```python
from build123d import *

# Parameters (mm, degrees)
SKETCH1_R           = 1.35
BOSS_EXTRUDE1_DEPTH = 3
SKETCH2_R           = 2
CUT_EXTRUDE1_DEPTH  = 110.604839186
FILLET1_R           = 2


with BuildPart() as part:
    # Sketch1 → Boss-Extrude1 (new body)
    with BuildSketch(Plane.XY):
        Polygon((78.713203436, 49.493203436), (57.5, 28.28), (57.5, -28.28), (78.713203436, -49.493203436), (51.993203436, -76.213203436), (30.78, -55), (-30.78, -55), (-51.993203436, -76.213203436), (-78.713203436, -49.493203436), (-57.5, -28.28), (-57.5, 28.28), (-78.713203436, 49.493203436), (-51.993203436, 76.213203436), (-30.78, 55), (30.78, 55), (51.993203436, 76.213203436), align=None)
        with Locations((29, -24.5)):
            Circle(SKETCH1_R, mode=Mode.SUBTRACT)
        with Locations((29, 24.5)):
            Circle(SKETCH1_R, mode=Mode.SUBTRACT)
        with Locations((-29, -24.5)):
            Circle(SKETCH1_R, mode=Mode.SUBTRACT)
        with Locations((-29, 24.5)):
            Circle(SKETCH1_R, mode=Mode.SUBTRACT)
    extrude(amount=BOSS_EXTRUDE1_DEPTH)

    # Sketch2 → Cut-Extrude1 (cut, through all)
    with BuildSketch(Plane.XY.offset(3)):
        with Locations((43.079339828, 53.30726189)):
            Circle(SKETCH2_R)
        with Locations((53.685941546, 63.913863607)):
            Circle(SKETCH2_R)
        with Locations((55.80726189, 40.579339828)):
            Circle(SKETCH2_R)
        with Locations((66.413863607, 51.185941546)):
            Circle(SKETCH2_R)
        with Locations((-66.413863607, -51.185941546)):
            Circle(SKETCH2_R)
        with Locations((-55.80726189, -40.579339828)):
            Circle(SKETCH2_R)
        with Locations((-43.079339828, -53.30726189)):
            Circle(SKETCH2_R)
        with Locations((-53.685941546, -63.913863607)):
            Circle(SKETCH2_R)
        with Locations((-53.479114875, 64.120690278)):
            Circle(SKETCH2_R)
        with Locations((-42.872513158, 53.51408856)):
            Circle(SKETCH2_R)
        with Locations((-55.600435219, 40.786166499)):
            Circle(SKETCH2_R)
        with Locations((-66.207036937, 51.392768217)):
            Circle(SKETCH2_R)
        with Locations((55.600435219, -40.786166499)):
            Circle(SKETCH2_R)
        with Locations((42.872513157, -53.51408856)):
            Circle(SKETCH2_R)
        with Locations((66.207036937, -51.392768217)):
            Circle(SKETCH2_R)
        with Locations((53.479114875, -64.120690278)):
            Circle(SKETCH2_R)
        with BuildLine():
            Line((-38.5, 17.5), (-38.5, -17.5))
            ThreePointArc((-38.5, -17.5), (-45.5, -24.5), (-52.5, -17.5))
            Line((-52.5, -17.5), (-52.5, 17.5))
            ThreePointArc((-52.5, 17.5), (-45.5, 24.5), (-38.5, 17.5))
        make_face()
        with BuildLine():
            Line((38.5, 17.5), (38.5, -17.5))
            ThreePointArc((38.5, -17.5), (45.5, -24.5), (52.5, -17.5))
            Line((52.5, -17.5), (52.5, 17.5))
            ThreePointArc((52.5, 17.5), (45.5, 24.5), (38.5, 17.5))
        make_face()
    extrude(amount=-CUT_EXTRUDE1_DEPTH, mode=Mode.SUBTRACT)

    # Fillet1
    fillet1_edges = [part.edges().sort_by_distance(p)[0] for p in [
        (78.713203436, -49.493203436, 1.5),
        (51.993203436, -76.213203436, 1.5),
        (-51.993203436, -76.213203436, 1.5),
        (-78.713203436, -49.493203436, 1.5),
        (-78.713203436, 49.493203436, 1.5),
        (-51.993203436, 76.213203436, 1.5),
        (51.993203436, 76.213203436, 1.5),
        (78.713203436, 49.493203436, 1.5),
    ]]
    fillet(fillet1_edges, radius=FILLET1_R)


solid = part.part
```
Can you work these out from the model? Positions are in its coordinate system, mm. A direction names the side the tool comes from. Round coordinates to 2 decimals unless told otherwise and drop trailing zeros. Loops run counter-clockwise (first coordinate to the right, second up) from the corner with the lowest first, then second, coordinate; pieces in that order, holes last. Notation, with made-up numbers: M 88.5,66.25 L 112.5,66.25 A25 cw 112.5,86.25 Z; hole C 4,22 d5. An arc over 180 degrees is marked long. Answer as a JSON object with one key per item and string values. Group by question number.
Q1. Imagine slicing it at A-A, the plane y = 1. Please give me the cut outline in (x, z), then the cut area to 3 significant figures.
Q2. Imagine slicing it at B-B, the plane x = 6.5. Please give me the cut outline in (y, z), then the cut area to 3 significant figures.
Q3. On a 3-axis mill with a long thin cutter (end or side, diameter ignored), from which of +Z, -Z, +X, -X, +Y, -Y can I reach the whole of each face in a straight line? I mean faces 1 (the cylindrical face through (45.65, 24.5, 1.52)), 2 (the flat face through (-67.26, 38.04, 1.48)), 3 (the flat face through (-40.54, -64.76, 1.48)), 4 (the flat face through (40.54, 64.76, 1.48)). Say none if no direction works.
Q4. Will these pins go through, and if not, where does the flat tip stop? pin 1 (1 mm diameter, centred on y = 31, z = 2.5, fed in from +X); pin 2 (0.9 mm diameter, centred on y = 3.5, z = 1.5, fed in from +X); pin 3 (1.5 mm diameter, centred on x = 9, z = 1, fed in from -Y).
Q5. Please list where these lines run through material, in increasing order: L1, parallel to X at y = -14, z = 0.9; L2, parallel to Y at x = 29, z = 1; L3, parallel to Y at x = 65, z = 2.1.
Q6. We'd pull the mould along Y, two halves only. Please class faces 5 (the flat face through (1, 1, 3)), 6 (the cylindrical face through (55.327, -64.887, 1.521)), 7 (the flat face through (-40.82, 65.04, 1.48)): +Y half, -Y half, draft (parallel to the pull), parting line (faces both ways), or undercut.
Q7. Imagine slicing it at C-C, the plane z = 1.2. Count the separate pieces of the cut face and the enclosed holes in it, then the cut area to 3 significant figures.
Findings:
{
 "1": {"outline": "M -57.5,0 L -52.5,0 L -52.5,3 L -57.5,3 Z; M -38.5,0 L 38.5,0 L 38.5,3 L -38.5,3 Z; M 52.5,0 L 57.5,0 L 57.5,3 L 52.5,3 Z", "area": "261 mm2"},
 "2": {"outline": "M -55,0 L 55,0 L 55,3 L -55,3 Z", "area": "330 mm2"},
 "3": {"face 1": "+Z, -Z", "face 2": "+Z, -Z, -X", "face 3": "+Z, -Z, -Y", "face 4": "+Z, -Z, +Y"},
 "4": {"pin 1": "stops at x = 60.72", "pin 2": "stops at x = 57.5", "pin 3": "stops at y = -55"},
 "5": {"L1": "x = -57.5 to -52.5, -38.5 to 38.5, 52.5 to 57.5", "L2": "y = -55 to -25.85, -23.15 to 23.15, 25.85 to 55", "L3": "y = -63.21 to -52.99, -49.8 to -35.78, 35.78 to 49.77, 52.6 to 63.21"},
 "6": {"face 5": "draft", "face 6": "undercut", "face 7": "+Y half"},
 "7": {"separate pieces": "1", "enclosed holes": "22", "area": "14,200 mm2"}
}
